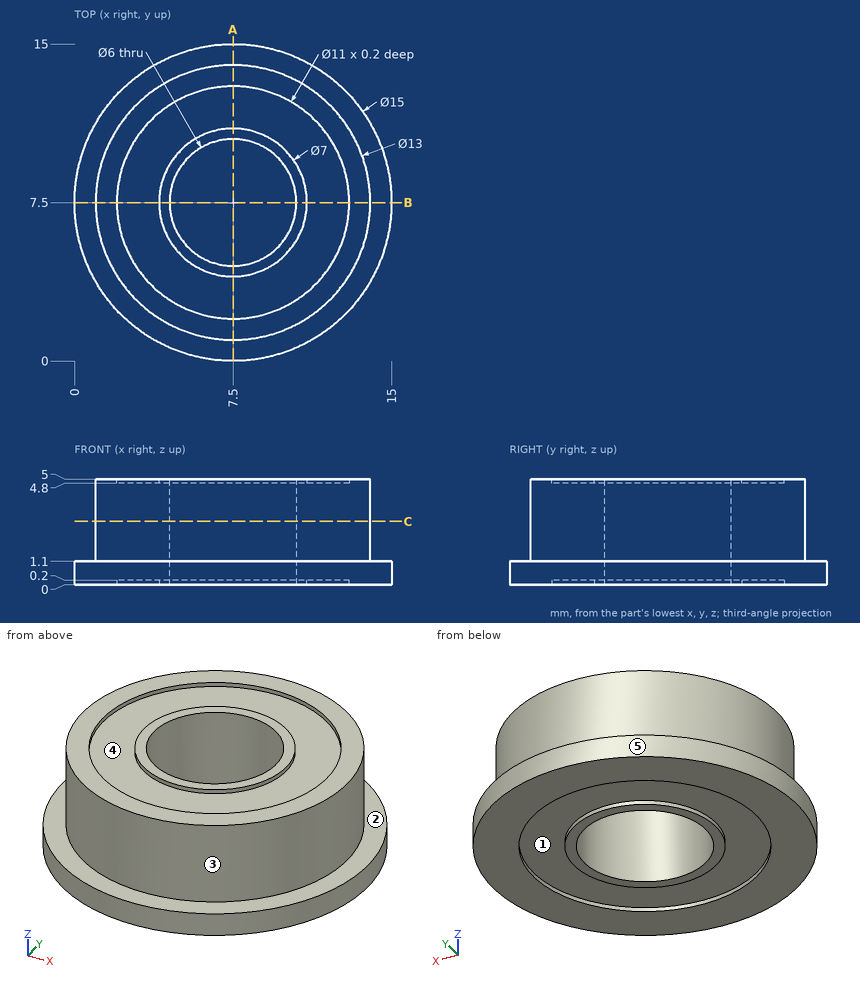
Study the drawing (mm; zero at the part's minimum x, y, z) and answer. A direction names the side the tool comes from. Give positions to 0.01 mm unless a question says otherwise; leave off trailing zeros. Loops run counter-clockwise (first coordinate to the right, second up) from the corner with the lowest first, then second, coordinate; pieces in that order, holes last. Notation, with made-up numbers: (7, 35.25) -> (17, 35.25) arc R27 ccw to (17, 69.25) -> close; hole circle Ø4 at (11, -3.5). An arc over 180 degrees is marked (long way). Use a Markdown table: item, result. Add a question column.
1) Which of the six approach directions +Z, -Z, +X, -X, +Y, -Y give full straight-line access (tool end or side, diameter ignored) to the marked faces 4 and 5?
2) The part is cut by section A-A, the plane x = 7.5. Determine the outline of the cut face in (y, z), plus the area to 3 significant figures.
3) The part is cut by section C-C, the plane z = 3. Determine the outline of the cut face in (x, y).
4) For a pull along X with two mould halves and no side action, classify the marked faces 1, 2 and 3 as +X half, -X half, draft (parallel to the pull), parting line (faces both ways), or undercut.
5) Each of these flat-tipped pins is pushed along its axis until it touches: P1, Ø3, axis at y = 3, z = 1.5, coming from the +X side; P2, Ø1, axis at y = 13, z = 1, coming from the -X side; P3, Ø1, axis at y = 8.5, z = 3.5, coming from the +X side. Where does it stop, or does it pass through?
6) Consider line 1 along Y through (x, z) = (7.5, 0.1); line 2 along Y through (x, z) = (7.5, 4.9); line 3 along Y through (x, z) = (7.5, 1.85). Determine where each line is inside the solid, lowest interval first.
Reported:
| question | item | result |
|---|---|---|
| 1 | face 4 | +Z |
| 1 | face 5 | +Z, -Z |
| 2 | outline | (0, 0) -> (2, 0) -> (2, 0.2) -> (4, 0.2) -> (4, 0) -> (4.5, 0) -> (4.5, 5) -> (4, 5) -> (4, 4.8) -> (2, 4.8) -> (2, 5) -> (1, 5) -> (1, 1.1) -> (0, 1.1) -> close; (10.5, 0) -> (11, 0) -> (11, 0.2) -> (13, 0.2) -> (13, 0) -> (15, 0) -> (15, 1.1) -> (14, 1.1) -> (14, 5) -> (13, 5) -> (13, 4.8) -> (11, 4.8) -> (11, 5) -> (10.5, 5) -> close |
| 2 | area | 35.6 mm^2 |
| 3 | outline | circle Ø13 at (7.5, 7.5); hole circle Ø6 at (7.5, 7.5) |
| 4 | face 1 | undercut |
| 4 | face 2 | draft |
| 4 | face 3 | parting line |
| 5 | P1 | stops at x = 14.35 |
| 5 | P2 | stops at x = 1.91 |
| 5 | P3 | stops at x = 13.98 |
| 6 | line 1 | y = 0 to 2, 4 to 4.5, 10.5 to 11, 13 to 15 |
| 6 | line 2 | y = 1 to 2, 4 to 4.5, 10.5 to 11, 13 to 14 |
| 6 | line 3 | y = 1 to 4.5, 10.5 to 14 |
